Model file for the job. Use its own axes, mm. A direction names the side the tool comes from. Round coordinates to 2 decimals unless told otherwise and drop trailing zeros. Order: outer loops, then holes, each group sorted by start corner. A loop starts at its lowest first (then second) coordinate and runs counter-clockwise, first axis right, second up. Notation, with made-up numbers: (3, 62) -> (47, 62) arc R9 ccw to (47, 74) -> close; hole circle Ø9 at (82, 5.25). An arc over 180 degrees is marked (long way). Answer as CSV lines item,"result".
```python
from build123d import *

# Parameters (mm, degrees)
F0_R     = 1.5
F1_DEPTH = 2.5
F2_R     = 5


with BuildPart() as f1:
    # F0 (on Front) → F1 (new body)
    with BuildSketch(Plane.XZ):
        Polygon((14, 10), (14, 35), (-14, 35), (-14, 10), (-25, 10), (-25, -35), (25, -35), (25, 10), align=None)
        with Locations((0, -28)):
            Circle(F0_R, mode=Mode.SUBTRACT)
        with Locations((0, 7.5)):
            Circle(F0_R, mode=Mode.SUBTRACT)
        with Locations((0, 27.5)):
            Circle(F0_R, mode=Mode.SUBTRACT)
    extrude(amount=F1_DEPTH)

    # F2
    f2_edges = [f1.edges().sort_by_distance(p)[0] for p in [
        (-14, -1.25, 10),
        (-25, -1.25, 10),
        (14, -1.25, 10),
        (25, -1.25, 10),
        (-25, -1.25, -35),
        (25, -1.25, -35),
        (14, -1.25, 35),
        (-14, -1.25, 35),
    ]]
    fillet(f2_edges, radius=F2_R)


solid = f1.part
```
Q1. Mould opens along X. For faces 1 (the cylindrical face through (15, -1, 12)), 2 (the flat face through (0, -1, 35)), 3 (the cylindrical face through (0, -1, 6)) say: +X half, -X half, draft (parallel to the pull), parting line (faces both ways), or undercut.
Checks:
face 1,"+X half"
face 2,"draft"
face 3,"undercut"
Q2. Tool access for faces 4 (the flat face through (14, -1, 22)), 5 (the cylindrical face through (24, -1, -33)): list every direction of +Z, -Z, +X, -X, +Y, -Y with a clear straight run to the whole face (end or side of a thin tool).
Checks:
face 4,"+Z, +X, +Y, -Y"
face 5,"-Z, +X, +Y, -Y"
Q3. Wall check: L1, parallel to Z at x = 0, y = -1.7; L2, parallel to Z at x = 19, y = -0.3; L3, parallel to X at y = -1.6, z = 22. Give the ranges that are in metal, low to high. Write a range as [from, to].
Checks:
L1,"[-35, -29.5], [-26.5, 6], [9, 26], [29, 35]"
L2,"[-35, 10]"
L3,"[-14, 14]"
Q4. Saw through at D-D (z = -28). Write the cut outline in (x, y).
Checks:
outline,"(-25, -2.5) -> (-1.5, -2.5) -> (-1.5, 0) -> (-25, 0) -> close; (1.5, -2.5) -> (25, -2.5) -> (25, 0) -> (1.5, 0) -> close"
Q5. Saw through at C-C (y = -1.25). Write the cut outline in (x, z), plus the area to 3 significant figures.
Checks:
outline,"(-25, -30) arc R5 ccw to (-20, -35) -> (20, -35) arc R5 ccw to (25, -30) -> (25, 5) arc R5 ccw to (20, 10) -> (19, 10) arc R5 cw to (14, 15) -> (14, 30) arc R5 ccw to (9, 35) -> (-9, 35) arc R5 ccw to (-14, 30) -> (-14, 15) arc R5 cw to (-19, 10) -> (-20, 10) arc R5 ccw to (-25, 5) -> close; hole circle Ø3 at (0, -28); hole circle Ø3 at (0, 7.5); hole circle Ø3 at (0, 27.5)"
area,"2,910 mm²"
Q6. Flat gauge pins, fed straight in: pin 1 (1.1 mm diameter, centred on x = 19.5, y = -2, fed in from +Z); pin 2 (2.5 mm diameter, centred on x = 0, z = 27.5, fed in from -Y); pin 3 (0.8 mm diameter, centred on y = -1.5, z = 25, fed in from -X). Where does each tip first touch, or does it go through?
Checks:
pin 1,"z = 10"
pin 2,"through"
pin 3,"x = -14"
Q7. Saw through at B-B (x = 0). Write the cut outline in (y, z), plus the area to 4 significant figures.
Checks:
outline,"(-2.5, -35) -> (0, -35) -> (0, -29.5) -> (-2.5, -29.5) -> close; (-2.5, -26.5) -> (0, -26.5) -> (0, 6) -> (-2.5, 6) -> close; (-2.5, 9) -> (0, 9) -> (0, 26) -> (-2.5, 26) -> close; (-2.5, 29) -> (0, 29) -> (0, 35) -> (-2.5, 35) -> close"
area,"152.5 mm²"
Q8. Saw through at A-A (z = 27.5). Write the cut outline in (x, y).
Checks:
outline,"(-14, -2.5) -> (-1.5, -2.5) -> (-1.5, 0) -> (-14, 0) -> close; (1.5, -2.5) -> (14, -2.5) -> (14, 0) -> (1.5, 0) -> close"
